```python
from build123d import *

# Parameters (mm, degrees)
SKETCH_1_R            = 105
EXTRUDE_359_DEPTH     = 3
CUT_EXTRUDE_769_DEPTH = 149.522725534
SKETCH_6_W            = 32
SKETCH_6_H            = 58
CUT_EXTRUDE_989_DEPTH = 149.522725534


with BuildPart() as part:
    # 草图1 → Extrude 359 (new body)
    with BuildSketch(Plane(origin=(0, 0, 0), x_dir=(1, 0, 0), z_dir=(0, 1, 0))):
        with Locations(Location((0, 0, 0), (0, 0, 270))):
            Circle(SKETCH_1_R)
    extrude(amount=EXTRUDE_359_DEPTH)

    # 草图5 → Cut-Extrude 769 (cut, through all)
    with BuildSketch(Plane(origin=(0, 3, 0), x_dir=(1, 0, 0), z_dir=(0, 1, 0))):
        with BuildLine():
            Line((-60, -20.5), (-102.979366865, -20.5))
            ThreePointArc((-102.979366865, -20.5), (-88.172313056, -57.014412304), (-60.948748962, -85.5))
            Line((-60.948748962, -85.5), (-60, -85.5))
            Line((-60, -85.5), (-60, -20.5))
        make_face()
        with BuildLine():
            ThreePointArc((60.948748962, -85.5), (88.172313056, -57.014412304), (102.979366865, -20.5))
            Line((102.979366865, -20.5), (60, -20.5))
            Line((60, -20.5), (60, -85.5))
            Line((60, -85.5), (60.948748962, -85.5))
        make_face()
    extrude(amount=-CUT_EXTRUDE_769_DEPTH, mode=Mode.SUBTRACT)

    # 草图6 → Cut-Extrude 989 (cut, through all)
    with BuildSketch(Plane(origin=(0, 3, 0), x_dir=(1, 0, 0), z_dir=(0, 1, 0))):
        with Locations((0, 67)):
            Rectangle(SKETCH_6_W, SKETCH_6_H)
    extrude(amount=-CUT_EXTRUDE_989_DEPTH, mode=Mode.SUBTRACT)


solid = part.part
```
Check sheet for the modelled part. Datum: model origin and axes. Units: mm. Give positions to 0.01 mm unless a question says otherwise; leave off trailing zeros. Order: outer loops, then holes, each group sorted by start corner. A loop starts at its lowest first (then second) coordinate and runs counter-clockwise, first axis right, second up. Notation, with made-up numbers: (-23, 8) -> (22, 8) arc R11 cw to (22, 26) -> close; hole circle Ø2 at (15.25, -11). An arc over 180 degrees is marked (long way). Use CSV: the item, a comma, the result in double quotes. Start each with the question number.
1) Sectioned sample at D-D, the plane z = 90.5. Record the boundary of the cut face in (x, y), plus the area to 3 significant figures.
2) Sectioned sample at A-A, the plane x = 0. Record the boundary of the cut face in (y, z).
3) Go/stop test with flat-tipped pins: P1, Ø4, axis at x = -17, z = -20.5, coming from the -Y side; P2, Ø0.9, axis at y = 2, z = 65, coming from the +X side; P3, Ø0.5, axis at x = 60, y = 1.5, coming from the -Z side. Record where each tip stops, or that it passes through.
4) Sectioned sample at B-B, the plane y = 2.2. Record the boundary of the cut face in (x, z).
5) Material ranges on line 1 (X direction, y = 0.3, z = 82); line 2 (X direction, y = 1.1, z = -61); line 3 (X direction, y = 1.95, z = -51.5), recorded low to high. Write a range as from..to.
6) Sectioned sample at C-C, the plane z = -86. Record the boundary of the cut face in (x, y).
Recorded:
1,outline,"(-53.24, 0) -> (53.24, 0) -> (53.24, 3) -> (-53.24, 3) -> close"
1,area,"319 mm2"
2,outline,"(0, -105) -> (3, -105) -> (3, -96) -> (0, -96) -> close; (0, -38) -> (3, -38) -> (3, 105) -> (0, 105) -> close"
3,P1,"y = 0"
3,P2,"x = 60"
3,P3,"z = -86.34"
4,outline,"(-102.98, 20.5) arc R105 ccw (long way) to (102.98, 20.5) -> (60, 20.5) -> (60, 85.5) -> (60.95, 85.5) arc R105 ccw to (-60.95, 85.5) -> (-60, 85.5) -> (-60, 20.5) -> close; hole (-16, -96) -> (16, -96) -> (16, -38) -> (-16, -38) -> close"
5,line 1,"-60..60"
5,line 2,"-85.46..-16, 16..85.46"
5,line 3,"-91.5..-16, 16..91.5"
6,outline,"(-60.24, 0) -> (-16, 0) -> (-16, 3) -> (-60.24, 3) -> close; (16, 0) -> (60.24, 0) -> (60.24, 3) -> (16, 3) -> close"
